Source: three-view drawing plus pictorial views. Frame: mm from the lowest corner of the part. Coordinates: 2 decimals unless noted, no trailing zeros. Write each loop counter-clockwise with the first axis right and the second up, starting at its lowest first coordinate (ties: lowest second). Pieces come first, ordered by that corner, then holes. Notation, with made-up numbers: M -2.5,-3 L 28.5,-3 A14 ccw 28.5,11 Z; hole C 16.5,-18.5 d7. An arc over 180 degrees is marked long. Write item = value, one per line. Start each with the question number.
Item 1: Section B-B on y = 8. Output: boundary loops of the cut face in (x, z).
Item 2: Ray query, L1, parallel to Y at x = 8.5, z = 1.5 (1 decimal); L2, parallel to Y at x = 14, z = 0.8 (1 decimal); L3, parallel to Y at x = 13.25, z = 2. Return the intervals inside material, ascending. Write a range as [from, to].
Item 3: First-contact query: pin 1 Ø2 at (x, y) = (8, 14) entering from +Z; pin 2 Ø1.4 at (x, y) = (13.2, 5) entering from +Z; pin 3 Ø1 at (y, z) = (6.5, 2) entering from +X. Flat tips, straight axial feed; report the tip coordinate or a pass-through.
Item 4: Section C-C on z = 2.05. Output: boundary loops of the cut face in (x, y).
Item 5: Pull-direction query (Y, two-part tool) for the marked faces 1, 2 and 3; classes: +Y half, -Y half, draft (parallel to the pull), parting line (faces both ways), or undercut.
Item 6: Section A-A on x = 8. Output: boundary loops of the cut face in (y, z).
Item 7: Section D-D on y = 5. Output: boundary loops of the cut face in (x, z), plus the area to 3 significant figures.
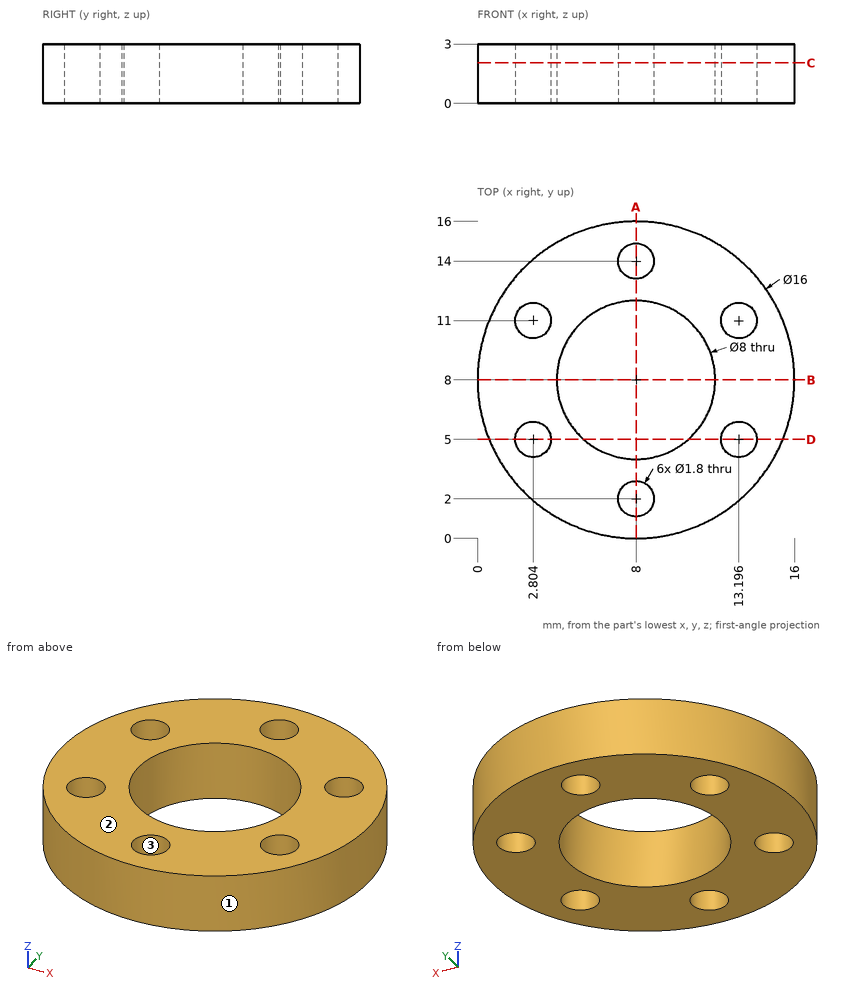
Responses:
q1.outline = M 0,0 L 4,0 L 4,3 L 0,3 Z; M 12,0 L 16,0 L 16,3 L 12,3 Z
q2.L1 = [0, 1.3], [2.7, 4], [12, 13.3], [14.7, 16]
q2.L2 = [2.7, 4.6], [5.4, 10.6], [11.4, 13.3]
q2.L3 = [1.96, 4.1], [5.9, 10.1], [11.9, 14.04]
q3.pin_1 = 3
q3.pin_2 = through
q3.pin_3 = 15.94
q4.outline = C 8,8 d16; hole C 2.8,5 d1.8; hole C 2.8,11 d1.8; hole C 8,8 d8; hole C 8,2 d1.8; hole C 8,14 d1.8; hole C 13.2,5 d1.8; hole C 13.2,11 d1.8
q5.face_1 = parting line
q5.face_2 = draft
q5.face_3 = undercut
q6.outline = M 0,0 L 1.1,0 L 1.1,3 L 0,3 Z; M 2.9,0 L 4,0 L 4,3 L 2.9,3 Z; M 12,0 L 13.1,0 L 13.1,3 L 12,3 Z; M 14.9,0 L 16,0 L 16,3 L 14.9,3 Z
q7.outline = M 0.58,0 L 1.9,0 L 1.9,3 L 0.58,3 Z; M 3.7,0 L 5.35,0 L 5.35,3 L 3.7,3 Z; M 10.65,0 L 12.3,0 L 12.3,3 L 10.65,3 Z; M 14.1,0 L 15.42,0 L 15.42,3 L 14.1,3 Z
q7.area = 17.8 mm²
